Autodesk Inventor part; units mm, degrees
ref_plane "YZ Plane" through (0, 0, 0) normal (1, 0, 0) x (0, 1, 0)
ref_plane "XZ Plane" through (0, 0, 0) normal (0, 1, 0) x (-1, 0, 0)
ref_plane "XY Plane" through (0, 0, 0) normal (0, 0, 1) x (1, 0, 0)
sketch "Sketch1" plane through (0, 0, 0) normal (0, 1, 0) x (-1, 0, 0)
  line L0 (21.9355, 25.495) -> (-52.0645, 25.495)
  line L1 (-52.0645, 25.495) -> (-52.0645, -94.005)
  line L2 (-52.0645, -94.005) -> (21.9355, -94.005)
  line L3 (21.9355, -94.005) -> (21.9355, 25.495)
  point P0 (0, 0)
  dimension "d0" = 119.5
  dimension "d1" = 74
extrude "Extrusion1" add sketch "Sketch1" against normal blind 3
sketch "Sketch2" plane through (0, 0, 0) normal (0, 1, 0) x (1, 0, 0)
  line L0 (-13.9355, -16.995) -> (-13.9355, 85.505)
  line L1 (-13.9355, 85.505) -> (47.0645, 85.505)
  line L2 (-21.9355, 94.005) -> (52.0645, 94.005)
  line L3 (47.0645, 85.505) -> (47.0645, -16.995)
  line L4 (47.0645, -16.995) -> (-13.9355, -16.995)
  line L5 (-21.9355, -25.495) -> (52.0645, -25.495)
  line L6 (-21.9355, 94.005) -> (-21.9355, -25.495)
  line L7 (52.0645, -25.495) -> (52.0645, 94.005)
  point P0 (0, 0)
  dimension "d4" = 8.5
  dimension "d5" = 8.5
  dimension "d6" = 8
  dimension "d7" = 5
extrude "Extrusion2" cut sketch "Sketch2" against normal blind 3 contours L0 L1 L3 L4
sketch "Sketch7" plane through (0, -3, 0) normal (0, -1, 0) x (1, 0, 0)
  line L0 (52.0645, 25.495) -> (-21.9355, 25.495)
  line L1 (52.0645, 25.495) -> (52.0645, 21.995)
  line L2 (52.0645, -94.005) -> (52.0645, 25.495)
  line L3 (52.0645, 21.995) -> (-21.9355, 21.995)
  line L4 (-21.9355, 21.995) -> (-21.9355, 25.495)
  line L5 (-21.9355, 25.495) -> (52.0645, 25.495)
  line L6 (52.0645, -94.005) -> (52.0645, -90.505)
  line L7 (52.0645, -90.505) -> (-21.9355, -90.505)
  line L8 (-21.9355, -90.505) -> (-21.9355, -94.005)
  line L9 (-21.9355, -94.005) -> (52.0645, -94.005)
  point P0 (0, 0)
  point P1 (-21.9355, 25.495)
  dimension "d82" = 3.5
  dimension "d83" = 74
  dimension "d84" = 3.5
  dimension "d107" = 74
extrude "Extrusion7" add sketch "Sketch7" along normal blind 8.5
sketch "Sketch8" plane through (52.0645, 0, 25.495) normal (1, 0, 0) x (0, 0, -1)
  line L0 (3.5, -3) -> (3.5, -11.5)
  line L1 (3.5, -5.75) -> (5, -7.25)
  line L2 (5, -7.25) -> (3.5, -8.75)
  line L3 (116, -3) -> (3.5, -3)
  line L4 (116, -3) -> (116, -11.5)
  line L5 (116, -5.75) -> (114.5, -7.25)
  line L6 (114.5, -7.25) -> (116, -8.75)
  point P0 (25.495, 0)
  dimension "d87" = 45
  dimension "d88" = 1.5
  dimension "d89" = 4.25
  dimension "d90" = 45
  dimension "d91" = 45
  dimension "d92" = 4.25
  dimension "d93" = 1.5
extrude "Extrusion8" add sketch "Sketch8" against normal blind 74
sketch "Sketch9" plane through (0, -11.5, 0) normal (0, -1, 0) x (1, 0, 0)
  line L0 (-21.9355, 25.495) -> (52.0645, 25.495)
  line L1 (10.0645, 25.495) -> (19.0645, 25.495)
  line L2 (19.0645, 25.495) -> (19.0645, 22.495)
  line L3 (10.0645, 22.495) -> (10.0645, 25.495)
  line L4 (52.0645, 21.995) -> (52.0645, 25.495)
  line L5 (-21.9355, 25.495) -> (-21.9355, 21.995)
  line L6 (10.0645, 22.495) -> (19.0645, 22.495)
  line L7 (52.0645, 21.995) -> (-21.9355, 21.995)
  point P0 (0, 0)
  dimension "d96" = 9
  dimension "d97" = 3
  dimension "d99" = 32
extrude "Extrusion9" add sketch "Sketch9" along normal blind 10 contours L0 L2 L6 L3
sketch "Sketch10" plane through (-21.9355, 0, 25.495) normal (0, 0, 1) x (1, 0, 0)
  circle A0 centre (36.5, -16.5) radius 1.5
  line L0 (41, -21.5) -> (32, -21.5)
  line L1 (32, -11.5) -> (32, -21.5)
  point P0 (21.9355, 0)
  dimension "d102" = 3
  dimension "d103" = 5
  dimension "d104" = 4.5
extrude "Extrusion10" cut sketch "Sketch10" against normal blind 10
properties part number "plate top"
Could you check a few things on this model? Use its own coordinates, in mm. A direction names the side the tool comes from. Round coordinates to 2 decimals unless told otherwise and drop trailing zeros. Order: outer loops, then holes, each group sorted by start corner. A loop starts at its lowest first (then second) coordinate and runs counter-clockwise, first axis right, second up.
(1) Imagine slicing it at B-B (z = -48). Write out the boundary of the cut face in (x, y), plus the area to 3 significant figures.
Response values:
outline: (-21.94, -3) - (-13.94, -3) - (-13.94, 0) - (-21.94, 0) - close; (47.06, -3) - (52.06, -3) - (52.06, 0) - (47.06, 0) - close
area: 39.0 mm2
(2) Imagine slicing it at C-C (y = -12.75). Write out the boundary of the cut face in (x, z) (1 decimal), plus the area to 3 significant figures.
Response values:
outline: (10.1, 22.5) - (19.1, 22.5) - (19.1, 25.5) - (10.1, 25.5) - close
area: 27.0 mm2
(3) Please list where these lines run through material, in increasing order: line 1 along Z through (x, y) = (-7.5, -1.25) (3 decimals); line 2 along Z through (x, y) = (2, -11) (3 decimals); line 3 along Y through (x, z) = (49.5, -26).
Response values:
line 1: z = -94.005 to -85.505, 16.995 to 25.495
line 2: z = -94.005 to -90.505, 21.995 to 25.495
line 3: y = -3 to 0
(4) I'm going to push flat-ended pins straight in: pin 1 (7 mm diameter, centred on x = 13, y = -18, fed in from -Z) (3 decimals); pin 2 (1.5 mm diameter, centred on y = -14, z = 24.5, fed in from +X); pin 3 (2.5 mm diameter, centred on y = -14.5, z = 24, fed in from -X). Where does each tip first touch, or does it pass through?
Response values:
pin 1: stops at z = 22.495
pin 2: stops at x = 19.06
pin 3: stops at x = 10.06
(5) Imagine slicing it at A-A (x = 30). Write out the boundary of the cut face in (y, z) (3 decimals).
Response values:
outline: (-11.5, -94.005) - (0, -94.005) - (0, -85.505) - (-3, -85.505) - (-3, -90.505) - (-5.75, -90.505) - (-7.25, -89.005) - (-8.75, -90.505) - (-11.5, -90.505) - close; (-11.5, 21.995) - (-8.75, 21.995) - (-7.25, 20.495) - (-5.75, 21.995) - (-3, 21.995) - (-3, 16.995) - (0, 16.995) - (0, 25.495) - (-11.5, 25.495) - close
(6) If we mould it in two halves opening along X, with no side actions, what happens to faces 6 (the flat face through (10.064, -16, 24)), 7 (the cylindrical face through (15.995, -16.049, 24.016)), 8 (the flat face through (16, -10, -90.505))? For each: released by +X, released by -X, zero draft, split by the parting line, or undercut.
Response values:
face 6: released by -X
face 7: undercut
face 8: zero draft
(7) Which directions (+Z, -Z, +X, -X, +Y, -Y) give clear straight access to the entire face, cutting with the end or side of a thin tool? Please do faces 1 (the flat face through (16, -4, -90.505)), 2 (the flat face through (16, -15, 22.495)), 3 (the flat face through (19.064, -16, 24)), 4 (the flat face through (16, -1, -85.505)), 5 (the flat face through (16, -10, 21.995)).
Response values:
face 1: +X, -X
face 2: -Z, +X, -X, -Y
face 3: +Z, -Z, +X, -Y
face 4: +Y, -Y
face 5: +X, -X, -Y
